Check sheet for the drawn part. Datum: minimum x, y, z corner. Units: mm. A direction names the side the tool comes from. Give positions to 0.01 mm unless a question says otherwise; leave off trailing zeros. Order: outer loops, then holes, each group sorted by start corner. A loop starts at its lowest first (then second) coordinate and runs counter-clockwise, first axis right, second up. Notation, with made-up numbers: (11.5, 50) -> (37.5, 50) arc R21 cw to (37.5, 86) -> close; hole circle Ø9 at (87, 0.25). An arc over 180 degrees is marked (long way). One line per question, with ' | ' between items. Start each with the question number.
Q1. Material ranges on probe 1 along Y at (x, z) = (20.5, 3.25); probe 2 along X at (y, z) = (18.5, 3.5); probe 3 along X at (y, z) = (5, 3.25), recorded low to high. Write a range as [from, to].
Q2. Go/stop test with a flat-tipped pin: pin 1 (12 mm diameter, centred on x = 28, y = 7, fed in from -Z). Record where the tip stops, or that it passes through.
Q3. Section check A-A on y = 22. Record the cut outline in (x, z).
Q4. Section check B-B on z = 3. Record the cut outline in (x, y), plus the area to 3 significant figures.
Q5. Mould release check, pull along X, two halves, no side actions. Record for the marked faces 3, 4, 5 and 6: released by +X, released by -X, zero draft, split by the parting line, or undercut.
Q6. Section check C-C on x = 53. Record the cut outline in (y, z), plus the area to 3 significant figures.
Q7. Access from +Z, -Z, +X, -X, +Y, -Y to the whole of each face (thin tool, end or side, straight path). Record for the marked faces 1 and 2.
Q8. Section check D-D on x = 3. Record the cut outline in (y, z), plus the area to 3 significant figures.
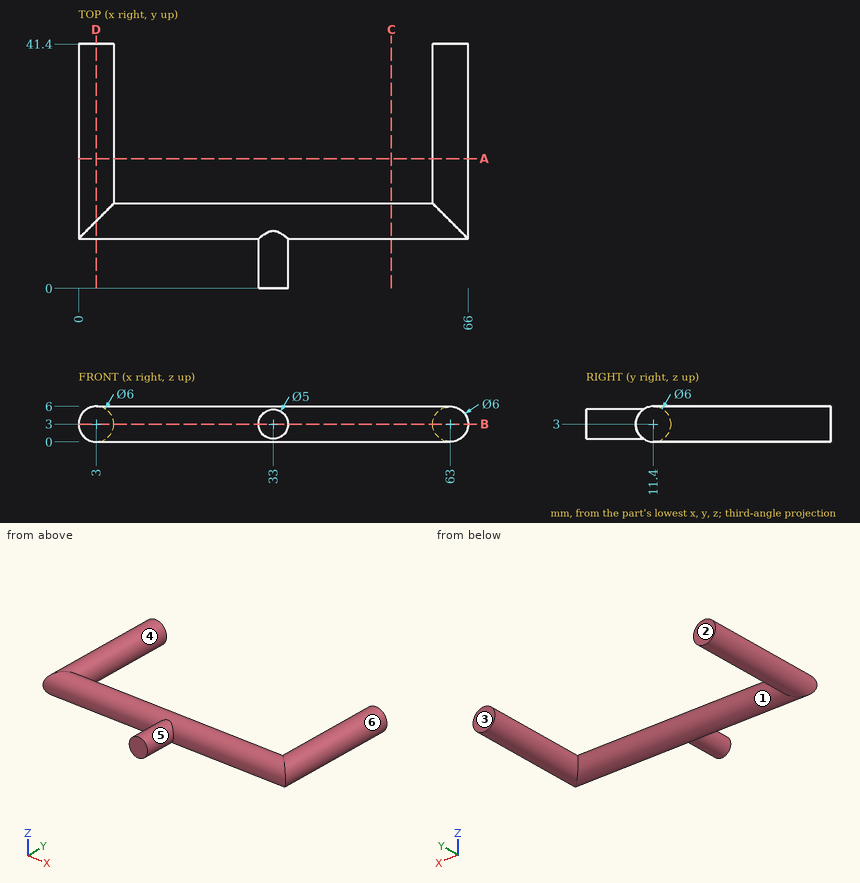
Filled in:
1) probe 1: [8.41, 14.39] | probe 2: [0.04, 5.96], [60.04, 65.96] | probe 3: [30.51, 35.49]
2) pin 1: z = 0
3) outline: circle Ø6 at (3, 3); circle Ø6 at (63, 3)
4) outline: (0, 8.4) -> (30.5, 8.4) -> (30.5, 0) -> (35.5, 0) -> (35.5, 8.4) -> (66, 8.4) -> (66, 41.4) -> (60, 41.4) -> (60, 14.4) -> (6, 14.4) -> (6, 41.4) -> (0, 41.4) -> close | area: 762 mm²
5) face 3: zero draft | face 4: undercut | face 5: split by the parting line | face 6: undercut
6) outline: circle Ø6 at (11.4, 3) | area: 28.3 mm²
7) face 1: none | face 2: +Z, -Z, +X, -X, +Y
8) outline: (11.4, 0) -> (41.4, 0) -> (41.4, 6) -> (11.4, 6) arc R3 ccw to start | area: 194 mm²
